Autodesk Inventor part; units mm, degrees
ref_plane "YZ Plane" through (0, 0, 0) normal (1, 0, 0) x (0, 1, 0)
ref_plane "XZ Plane" through (0, 0, 0) normal (0, 1, 0) x (-1, 0, 0)
ref_plane "XY Plane" through (0, 0, 0) normal (0, 0, 1) x (1, 0, 0)
sketch "Szkic1" plane through (0, 0, 0) normal (0, 0, 1) x (1, 0, 0)
  line L0 (-10.699, 18.8462) -> (5.301, 18.8462)
  line L1 (5.301, 18.8462) -> (5.301, -13.5538)
  line L2 (5.301, -13.5538) -> (-10.699, -13.5538)
  line L3 (-10.699, -13.5538) -> (-10.699, 18.8462)
  point P0 (0, 0)
  dimension "d0" = 16
  dimension "d1" = 32.4
extrude "Wyciągnięcie proste1" add sketch "Szkic1" along normal blind 10
sketch "Szkic2" plane through (-10.699, -13.5538, 0) normal (-1, 0, 0) x (0, 0, 1)
  line L0 (0, 0) -> (0, 32.4)
  line L1 (0, 0) -> (10, 0)
  line L2 (10, 32.4) -> (10, 0)
  line L3 (0, 32.4) -> (10, 32.4)
  line L4 (10, 32.4) -> (10, 0)
  circle A0 centre (10, 16.2) radius 6.05
  point P0 (0, 13.5538)
  dimension "d4" = 32.4
  dimension "d5" = 16.2
  dimension "d6" = 12.1
extrude "Wyciągnięcie proste2" cut sketch "Szkic2" against normal blind 13 contours A0 L2 | L2 A0
sketch "Szkic3" plane through (-10.699, -13.5538, 0) normal (-1, 0, 0) x (0, 0, 1)
  arc A0 (10, 22.25) -> (10, 10.15) centre (10, 16.2) ccw
  line L0 (10, 32.4) -> (10, 22.25)
  line L1 (0, 32.4) -> (10, 32.4)
  line L2 (0, 0) -> (0, 32.4)
  line L3 (0, 0) -> (10, 0)
  line L4 (10, 10.15) -> (10, 0)
  arc A1 (10, 24.275) -> (10, 8.125) centre (10, 16.2) ccw
  point P0 (0, 13.5538)
  dimension "d9" = 16.15
extrude "Wyciągnięcie proste3" cut sketch "Szkic3" against normal blind 7.15 contours A0 L4 A1 L0
extrude "Wyciągnięcie proste4" add sketch "Szkic3" against normal blind 3.3 contours A0 L4 A1 L0
sketch "Szkic6" plane through (5.301, -13.5538, 0) normal (1, 0, 0) x (0, 0, -1)
  arc A0 (-10, 8.125) -> (-10, 24.275) centre (-10, 16.2) ccw
  line L0 (0, 32.4) -> (0, 0)
  line L1 (0, 32.4) -> (-10, 32.4)
  line L2 (-10, 0) -> (-10, 32.4)
  line L3 (0, 0) -> (-10, 0)
  arc A1 (-10, 8.125) -> (-10, 24.275) centre (-10, 16.2) ccw
  point P0 (0, 13.5538)
extrude "Wyciągnięcie proste5" cut sketch "Szkic6" against normal blind 3.15 contours L2 A0
sketch "Szkic7" plane through (0, 0, 10) normal (0, 0, 1) x (1, 0, 0)
  line L0 (5.301, -5.4288) -> (2.151, -5.4288)
  line L1 (2.151, -5.4288) -> (2.151, -3.4038)
  line L2 (2.151, -3.4038) -> (-3.549, -3.4038)
  line L3 (-3.549, -3.4038) -> (-3.549, -5.4288)
  line L4 (-3.549, -5.4288) -> (-7.399, -5.4288)
  line L5 (-7.399, -3.4038) -> (-7.399, -5.4288)
  line L6 (-10.699, -3.4038) -> (-7.399, -3.4038)
  line L7 (-10.699, -3.4038) -> (-10.699, -13.5538)
  line L8 (-10.699, -13.5538) -> (5.301, -13.5538)
  line L9 (5.301, -13.5538) -> (5.301, -5.4288)
  line L10 (2.151, 10.7212) -> (5.301, 10.7212)
  line L11 (5.301, 10.7212) -> (5.301, 18.8462)
  line L12 (5.301, 18.8462) -> (-10.699, 18.8462)
  line L13 (-10.699, 18.8462) -> (-10.699, 8.6962)
  line L14 (-10.699, 8.6962) -> (-7.399, 8.6962)
  line L15 (-7.399, 10.7212) -> (-7.399, 8.6962)
  line L16 (-7.399, 10.7212) -> (-3.549, 10.7212)
  line L17 (-3.549, 10.7212) -> (-3.549, 8.6962)
  line L18 (-3.549, 8.6962) -> (2.151, 8.6962)
  line L19 (2.151, 8.6962) -> (2.151, 10.7212)
  point P0 (0, 0)
  point P1 (-0.699, -7.3538)
  point P2 (-0.699, 12.6462)
  dimension "d46" = 20
  dimension "d47" = 32.4
  dimension "d48" = 6.2
  dimension "d49" = 6.2
  dimension "d50" = 5.7
  dimension "d96" = 10
  dimension "d97" = 10
hole "Otwór3" at (-0.699, -7.3538, 10) at (-0.699, 12.6462, 10) direction (0, 0, -1) diameter 3 end through all
chamfer "Faza4" distance 1.5 angle 45 2 edges at (5.301, -13.5538, 5) (5.301, 18.8462, 5)
sketch "Szkic9" plane through (-10.699, -13.5538, 0) normal (-1, 0, 0) x (0, 0, 1)
  line L0 (10, 32.4) -> (10, 22.25)
  line L1 (0, 32.4) -> (10, 32.4)
  line L2 (0, 0) -> (0, 32.4)
  line L3 (0, 0) -> (10, 0)
  line L4 (10, 10.15) -> (10, 0)
  arc A0 (10, 22.25) -> (10, 10.15) centre (10, 16.2) ccw
  point P0 (0, 13.5538)
extrude "Wyciągnięcie proste7" add sketch "Szkic9" along normal blind 2
chamfer "Faza8" distance 1.5 angle 45 2 edges at (-12.699, -13.5538, 5) (-12.699, 18.8462, 5)
chamfer "Faza9" distance 1 angle 45 1 edges at (-12.699, 2.6462, 3.95)
sketch "Szkic10" plane through (0, 0, 10) normal (0, 0, 1) x (1, 0, 0)
  circle A0 centre (-0.699, -7.3538) radius 1.5
  line L0 (-12.699, -4.4038) -> (-11.699, -3.4038)
  line L1 (-12.699, -12.0538) -> (-12.699, -4.4038)
  line L2 (-11.199, -13.5538) -> (-12.699, -12.0538)
  line L3 (3.801, -13.5538) -> (-11.199, -13.5538)
  line L4 (5.301, -12.0538) -> (3.801, -13.5538)
  line L5 (5.301, -12.0538) -> (5.301, -5.4288)
  line L6 (5.301, -5.4288) -> (2.151, -5.4288)
  line L7 (2.151, -5.4288) -> (2.151, -3.4038)
  line L8 (2.151, -3.4038) -> (-3.549, -3.4038)
  line L9 (-3.549, -3.4038) -> (-3.549, -5.4288)
  line L10 (-3.549, -5.4288) -> (-7.399, -5.4288)
  line L11 (-7.399, -3.4038) -> (-7.399, -5.4288)
  line L12 (-11.699, -3.4038) -> (-7.399, -3.4038)
  line L13 (-11.699, 8.6962) -> (-12.699, 9.6962)
  line L14 (-7.399, 8.6962) -> (-11.699, 8.6962)
  line L15 (-7.399, 10.7212) -> (-7.399, 8.6962)
  line L16 (-7.399, 10.7212) -> (-3.549, 10.7212)
  line L17 (-3.549, 10.7212) -> (-3.549, 8.6962)
  line L18 (-3.549, 8.6962) -> (2.151, 8.6962)
  line L19 (2.151, 8.6962) -> (2.151, 10.7212)
  line L20 (2.151, 10.7212) -> (5.301, 10.7212)
  line L21 (5.301, 10.7212) -> (5.301, 17.3462)
  line L22 (3.801, 18.8462) -> (5.301, 17.3462)
  line L23 (3.801, 18.8462) -> (-11.199, 18.8462)
  line L24 (-12.699, 17.3462) -> (-11.199, 18.8462)
  line L25 (-12.699, 9.6962) -> (-12.699, 17.3462)
  circle A1 centre (-0.699, 12.6462) radius 1.5
  point P0 (0, 0)
  point P1 (-9.199, -9.5538)
  point P2 (-9.199, 14.8462)
  dimension "d106" = 4
  dimension "d107" = 4
  dimension "d108" = 3.5
  dimension "d109" = 3.5
hole "Otwór4" at (-9.199, -9.5538, 10) at (-9.199, 14.8462, 10) direction (0, 0, -1) diameter 3 end through all
properties part number "3DP_ABS_E3D_V6_Mount"
The model under review builds one solid part; all positions refer to its coordinate system, in mm. A direction names the side the tool comes from. Round coordinates to 2 decimals unless told otherwise and drop trailing zeros. Write each loop counter-clockwise with the first axis right and the second up, starting at its lowest first coordinate (ties: lowest second). Pieces come first, ordered by that corner, then holes. Notation, with made-up numbers: (20, 87.5) - (58, 87.5) arc R30 cw to (58, 113.5) - close; hole circle Ø7 at (49.25, 11). An arc over 180 degrees is marked (long way). Use one line per item in the form item = value.
Q1. Consider section B-B (z = 2.5). State the section outline as (x, y) points, and give its area (3 significant figures).
Answer key:
outline = (-12.7, -12.05) - (-11.2, -13.55) - (3.8, -13.55) - (5.3, -12.05) - (5.3, -0.35) - (2.15, -0.35) - (2.15, 5.64) - (5.3, 5.64) - (5.3, 17.35) - (3.8, 18.85) - (-11.2, 18.85) - (-12.7, 17.35) - close; hole circle Ø3 at (-9.2, -9.55); hole circle Ø3 at (-9.2, 14.85); hole (-7.4, -0.35) - (-3.55, -0.35) - (-3.55, 5.64) - (-7.4, 5.64) - close; hole circle Ø3 at (-0.7, -7.35); hole circle Ø3 at (-0.7, 12.65)
area = 509 mm2
Q2. Insertion check: pin 1 Ø2.5 at (x, y) = (-9.2, 14.85) entering from -Z. The pin has a flat end and moves straight along its axis. Give the tip position at first contact, or say it passes through.
Answer key:
pin_1 = through
Q3. Consider section D-D (z = 9). State how many separate pieces and enclosed holes the cut face has, and give its area (3 significant figures).
Answer key:
separate_pieces = 2
enclosed_holes = 4
area = 306 mm2
Q4. Draft analysis for pull direction Y (two halves, no side actions). For faces 4 (the flat face through (4.56, 18.09, 4.93)), 5 (the flat face through (5.301, 2.9, 1.6)), 6 (the conical face through (-11.87, 2.78, 3.78)), state which applies: +Y half, -Y half, draft (parallel to the pull), parting line (faces both ways), or undercut.
Answer key:
face_4 = +Y half
face_5 = draft
face_6 = undercut
Q5. For line 1 (X direction, y = -7.5, z = 3); line 2 (X direction, y = 6, z = 3.75); line 3 (X direction, y = 14, z = 8), list the stretches that pass through material, from the lowest coordinate up. Write a range as [from, to].
Answer key:
line_1 = [-12.7, -2.19], [0.79, 5.3]
line_2 = [-12.7, -7.4], [-3.55, 2.15]
line_3 = [-12.7, -10.44], [-7.96, -1.34], [-0.05, 5.3]
Q6. Consider section C-C (y = -5). State the section outline as (x, z) points.
Answer key:
outline = (-12.7, 0) - (5.3, 0) - (5.3, 7.4) - (2.15, 7.4) - (2.15, 10) - (-3.55, 10) - (-3.55, 7.4) - (-7.4, 7.4) - (-7.4, 10) - (-12.7, 10) - close
Q7. Consider section A-A (x = 0). State the section outline as (y, z) points.
Answer key:
outline = (-13.55, 0) - (-8.68, 0) - (-8.68, 10) - (-13.55, 10) - close; (-6.03, 0) - (11.32, 0) - (11.32, 10) - (8.7, 10) arc R6.05 cw to (-3.4, 10) - (-6.03, 10) - close; (13.97, 0) - (18.85, 0) - (18.85, 10) - (13.97, 10) - close
Q8. Tool access review of faces 1 (the flat face through (2.151, 2.1, 3.6)), 2 (the flat face through (-12.699, 2.9, 2.7)), 3 (the flat face through (-3.549, 3, 3)): name each direction out of +Z, -Z, +X, -X, +Y, -Y from which nothing blocks a thin tool from reaching the whole face with its end or side.
Answer key:
face_1 = +Z, +X
face_2 = +Z, -Z, -X, +Y, -Y
face_3 = +Z
